Verification items for the finished model (mm, model axes). Coordinates: 2 decimals unless noted, no trailing zeros. Write each loop counter-clockwise with the first axis right and the second up, starting at its lowest first coordinate (ties: lowest second). Pieces come first, ordered by that corner, then holes. Notation, with made-up numbers: M -12,46 L 29,46 A19 ccw 29,74 Z; hole C 77,32.25 d9. An arc over 180 degrees is marked long. One line per item, written item: value.
```python
from build123d import *

# Parameters (mm, degrees)
SKETCH_1_R      = 1.649999992
SKETCH_1_R_2    = 1.649999999
SKETCH_1_R_3    = 1.65
EXTRUDE_1_DEPTH = 3
FILLET_2_R      = 5
FILLET_3_R      = 5


with BuildPart() as part:
    # 草图1 → 凸台-拉伸1 (new body)
    with BuildSketch(Plane(origin=(0, 0, 0), x_dir=(1, 0, 0), z_dir=(0, 1, 0))):
        Polygon((-28.332706405, -6.664922467), (-16.332704755, -22.664921194), (7.667293339, -4.664918716), (7.664042293, -34.664767296), (27.664042293, -34.664767296), (27.664489855, 35.332983845), (-4.33270825, 11.335080057), align=None)
        with Locations(Location((17.667491748, 15.335232704, 0), (0, 0, 270))):
            Circle(SKETCH_1_R, mode=Mode.SUBTRACT)
        with Locations(Location((17.667491748, -4.664767296, 0), (0, 0, 270))):
            Circle(SKETCH_1_R, mode=Mode.SUBTRACT)
        with Locations(Location((17.667491748, -24.664767296, 0), (0, 0, 270))):
            Circle(SKETCH_1_R, mode=Mode.SUBTRACT)
        with Locations(Location((-6.332706828, -2.664920166, 0), (0, 0, 270))):
            Circle(SKETCH_1_R_2, mode=Mode.SUBTRACT)
        with Locations(Location((-14.332706205, -8.664920997, 0), (0, 0, 270))):
            Circle(SKETCH_1_R_3, mode=Mode.SUBTRACT)
    extrude(amount=EXTRUDE_1_DEPTH)

    # 圆角2
    fillet_2_edges = [part.edges().sort_by_distance(p)[0] for p in [
        (7.667293339, 1.5, 4.664918716),
    ]]
    fillet(fillet_2_edges, radius=FILLET_2_R)

    # 圆角3
    fillet_3_edges = [part.edges().sort_by_distance(p)[0] for p in [
        (27.664489855, 1.5, -35.332983845),
    ]]
    fillet(fillet_3_edges, radius=FILLET_3_R)


solid = part.part
```
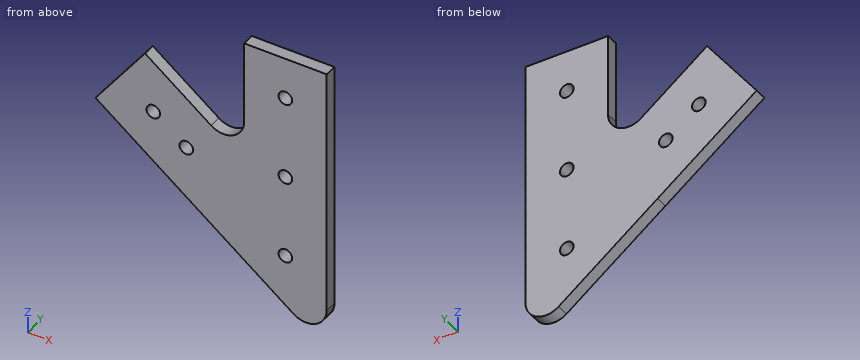
Item 1: Scan lines: line 1 (X direction, y = 0.95, z = 8); line 2 (Z direction, x = -7, y = 0.5); line 3 (X direction, y = 2.1, z = 25). Record each from-to range of solid material in increasing order.
The answers:
line 1: x = -27.33 to -15.84, -12.82 to 27.66
line 2: z = -9.33 to 1.16, 4.17 to 15.67
line 3: x = 7.67 to 16.05, 19.28 to 27.66
Item 2: Cross-section at A-A, the plane z = 17. Enter the section's corners in (x, y).
The answers:
outline: M -20.58,0 L -8.78,0 L -8.78,3 L -20.58,3 Z; M 7.67,0 L 27.66,0 L 27.66,3 L 7.67,3 Z
Item 3: Cross-section at C-C, the plane x = -22.5. Enter the section's corners in (y, z).
The answers:
outline: M 0,2.29 L 3,2.29 L 3,14.44 L 0,14.44 Z
Item 4: Go/stop test with flat-tipped pins: P1, Ø1.5, axis at y = 1, z = -15.5, coming from the -X side; P2, Ø1.5, axis at y = 2.5, z = 20, coming from the -X side; P3, Ø1, axis at x = 5, y = 1.5, coming from the -Z side. Record where each tip stops, or that it passes through.
The answers:
P1: stops at x = 0.22
P2: stops at x = -18.89
P3: stops at z = -18.71
Item 5: Cross-section at D-D, the plane z = 30.5. Enter the section's corners in (x, y).
The answers:
outline: M 7.66,0 L 27.66,0 L 27.66,3 L 7.66,3 Z
Item 6: Cross-section at B-B, the plane y = 1.55. Enter the section's corners in (x, z).
The answers:
outline: M -28.33,6.66 L 19.66,-29.33 A5 ccw 27.66,-25.33 L 27.66,34.66 L 7.66,34.66 L 7.67,14.67 A5 cw -0.33,10.67 L -16.33,22.66 Z; hole C -14.33,8.66 d3.3; hole C -6.33,2.66 d3.3; hole C 17.67,-15.34 d3.3; hole C 17.67,4.66 d3.3; hole C 17.67,24.66 d3.3
